```python
from build123d import *

# Parameters (mm, degrees)
MAIN_EXTRUSION_DEPTH         = 45
R_P_TITION_CIRCULAIRE1_DEPTH = 45
ESQUISSE2_R                  = 91.977766886
ESQUISSE2_R_2                = 40
GLOBAL_CIRCLE_DEPTH          = 1
CENTRAL_START                = 2
CENTRAL_FIXING_DEPTH         = 2
R_P_TITION_CIRCULAIRE2_COUNT = 8


# Read off the part's stored shape, not the designer's step: Répétition circulaire1
with BuildPart() as part:
    # Esquisse1 → Main Extrusion (new body)
    with BuildSketch(Plane.XY):
        with BuildLine():
            Line((57.667547326, 24.944747378), (84.602293038, 36.101484351))
            Line((84.602293038, 36.101484351), (85.750343335, 33.329845753))
            Line((85.750343335, 33.329845753), (58.815597623, 22.17310878))
            ThreePointArc((58.815597623, 22.17310878), (44, 0), (58.815597623, -22.17310878))
            Line((58.815597623, -22.17310878), (85.750343335, -33.329845753))
            Line((85.750343335, -33.329845753), (84.602293038, -36.101484351))
            Line((84.602293038, -36.101484351), (57.667547326, -24.944747378))
            ThreePointArc((57.667547326, -24.944747378), (41, 0), (57.667547326, 24.944747378))
        make_face()
    extrude(amount=MAIN_EXTRUSION_DEPTH)

    # Répétition circulaire1 outline → Répétition circulaire1 (add)
    with BuildSketch(Plane.XY):
        with BuildLine():
            Line((-84.202409209, -37.066889313), (-57.267663497, -25.91015234))
            ThreePointArc((-57.267663497, -25.91015234), (-31.112698372, -31.112698372), (-25.91015234, -57.267663497))
            Line((-25.91015234, -57.267663497), (-37.066889313, -84.202409209))
            Line((-37.066889313, -84.202409209), (-33.329845753, -85.750343335))
            Line((-33.329845753, -85.750343335), (-22.17310878, -58.815597623))
            ThreePointArc((-22.17310878, -58.815597623), (0, -44), (22.17310878, -58.815597623))
            Line((22.17310878, -58.815597623), (33.329845753, -85.750343335))
            Line((33.329845753, -85.750343335), (37.066889313, -84.202409209))
            Line((37.066889313, -84.202409209), (25.91015234, -57.267663497))
            ThreePointArc((25.91015234, -57.267663497), (31.112698372, -31.112698372), (57.267663497, -25.91015234))
            Line((57.267663497, -25.91015234), (84.202409209, -37.066889313))
            Line((84.202409209, -37.066889313), (84.602293038, -36.101484351))
            Line((84.602293038, -36.101484351), (57.667547326, -24.944747378))
            ThreePointArc((57.667547326, -24.944747378), (54.405305377, -23.327757675), (51.390283197, -21.286552275))
            ThreePointArc((51.390283197, -21.286552275), (28.991378029, -28.991378029), (21.286552275, -51.390283197))
            ThreePointArc((21.286552275, -51.390283197), (0, -41), (-21.286552275, -51.390283197))
            ThreePointArc((-21.286552275, -51.390283197), (-28.991378029, -28.991378029), (-51.390283197, -21.286552275))
            ThreePointArc((-51.390283197, -21.286552275), (-41, 0), (-51.390283197, 21.286552275))
            ThreePointArc((-51.390283197, 21.286552275), (-28.991378029, 28.991378029), (-21.286552275, 51.390283197))
            ThreePointArc((-21.286552275, 51.390283197), (0, 41), (21.286552275, 51.390283197))
            ThreePointArc((21.286552275, 51.390283197), (28.991378029, 28.991378029), (51.390283197, 21.286552275))
            ThreePointArc((51.390283197, 21.286552275), (54.405305377, 23.327757675), (57.667547326, 24.944747378))
            Line((57.667547326, 24.944747378), (84.602293038, 36.101484351))
            Line((84.602293038, 36.101484351), (84.202409209, 37.066889313))
            Line((84.202409209, 37.066889313), (57.267663497, 25.91015234))
            ThreePointArc((57.267663497, 25.91015234), (31.112698372, 31.112698372), (25.91015234, 57.267663497))
            Line((25.91015234, 57.267663497), (37.066889313, 84.202409209))
            Line((37.066889313, 84.202409209), (33.329845753, 85.750343335))
            Line((33.329845753, 85.750343335), (22.17310878, 58.815597623))
            ThreePointArc((22.17310878, 58.815597623), (0, 44), (-22.17310878, 58.815597623))
            Line((-22.17310878, 58.815597623), (-33.329845753, 85.750343335))
            Line((-33.329845753, 85.750343335), (-37.066889313, 84.202409209))
            Line((-37.066889313, 84.202409209), (-25.91015234, 57.267663497))
            ThreePointArc((-25.91015234, 57.267663497), (-31.112698372, 31.112698372), (-57.267663497, 25.91015234))
            Line((-57.267663497, 25.91015234), (-84.202409209, 37.066889313))
            Line((-84.202409209, 37.066889313), (-85.750343335, 33.329845753))
            Line((-85.750343335, 33.329845753), (-58.815597623, 22.17310878))
            ThreePointArc((-58.815597623, 22.17310878), (-44, 0), (-58.815597623, -22.17310878))
            Line((-58.815597623, -22.17310878), (-85.750343335, -33.329845753))
            Line((-85.750343335, -33.329845753), (-84.202409209, -37.066889313))
        make_face()
    extrude(amount=R_P_TITION_CIRCULAIRE1_DEPTH)

    # Esquisse2 → Global Circle (add)
    with BuildSketch(Plane.XY.offset(45)):
        with Locations(Location((0, 0, 0), (0, 0, 201.240037576))):
            Circle(ESQUISSE2_R)
        Circle(ESQUISSE2_R_2, mode=Mode.SUBTRACT)
    extrude(amount=GLOBAL_CIRCLE_DEPTH)

    # Esquisse3 → Central Fixing (add)
    with BuildSketch(Plane(origin=(0, 0, 45), x_dir=(-1, 0, 0), z_dir=(0, 0, -1)).offset(CENTRAL_START)):
        with BuildLine():
            Line((-5, 44.526610811), (-5, 0))
            Line((-5, 0), (-4, 0))
            Line((-4, 0), (-4, 5))
            Line((-4, 5), (4, 5))
            Line((4, 5), (4, 0))
            Line((4, 0), (5, 0))
            Line((5, 0), (5, 44.526610811))
            ThreePointArc((5, 44.526610811), (0, 44), (-5, 44.526610811))
        make_face()
    central_fixing = extrude(amount=-CENTRAL_FIXING_DEPTH)

    # Répétition circulaire2: Central Fixing ×8 about axis
    r_p_tition_circulaire2_axis = Axis((0, 0, 0), (0, 0, 1))
    for i in range(1, R_P_TITION_CIRCULAIRE2_COUNT):
        add(central_fixing.rotate(r_p_tition_circulaire2_axis, i * 360 / R_P_TITION_CIRCULAIRE2_COUNT))


solid = part.part
```
The model under review builds one solid part; all positions refer to its coordinate system, in mm. A direction names the side the tool comes from. Round coordinates to 2 decimals unless told otherwise and drop trailing zeros. Loops run counter-clockwise (first coordinate to the right, second up) from the corner with the lowest first, then second, coordinate; pieces in that order, holes last. Notation, with made-up numbers: (-20.5, 4) - (-4.5, 4) arc R19 cw to (-4.5, 9) - close; hole circle Ø5 at (71.5, 68.5). An arc over 180 degrees is marked (long way). Use a Markdown table: item, result. Add a question column.
Q1. For probe 1 along Y at (x, z) = (0, 45.45); probe 2 along Y at (x, z) = (-30.5, 35); probe 3 along Y at (x, z) = (35, 24), list the stretches that pass through material, from the lowest coordinate up.
Q2. Add section C-C (y = -75). State the section outline as (x, z) points.
Q3. Machinability: for faces 1 (the face through (0, -44, 22)), 2 (the face through (-70.55, 31.41, 22.18)), 3 (the face through (30.84, 31.39, 22.18)), 4 (the face through (31.41, 70.55, 22.18)), which of the approach directions +Z, -Z, +X, -X, +Y, -Y give a long, thin tool a straight path to every point of the face, cutting with its end or side? Answer none if there is none.
Q4. The part is to be moulded in two halves that separate along X. For faces 5 (the face through (44, 0, 22)), 6 (the face through (0, -41, 22)), 7 (the face through (-72.47, 27.83, 22.18)), 8 (the face through (-18, -40, 45)), say which applies: pulls with the +X half, pulls with the -X half, needs draft (parallel to the pull), parting line crosses it, or undercut.
Q5. Add section B-B (y = 9.5). State the section outline as (x, z) points.
Q6. Insertion check: pin 1 Ø4 at (y, z) = (-57.5, 36) entering from -X; pin 2 Ø1.5 at (x, y) = (49.5, -66.5) entering from -Z; pin 3 Ø2 at (y, z) = (-32, 43.5) entering from -X. Each pin has a flat end and moves straight along its axis. Give the tip position at first contact, or say it passes through.
Q7. Add section D-D (x = -73). State the section outline as (y, z) points, plus the area to 3 significant figures.
Q8. Add section A-A (x = -7.5). State the section outline as (y, z) points, plus the area to 3 significant figures.
Worked answers:
| question | item | result |
|---|---|---|
| 1 | probe 1 | -91.98 to -40, 40 to 91.98 |
| 1 | probe 2 | -78.92 to -68.35, -31.75 to -27.59, 27.59 to 31.75, 68.35 to 78.92 |
| 1 | probe 3 | -85.06 to -79.21, -27.96 to -24.46, 24.46 to 27.96, 79.21 to 85.06 |
| 2 | outline | (-53.24, 45) - (-33.26, 45) - (-33.26, 0) - (-28.88, 0) - (-28.88, 45) - (28.88, 45) - (28.88, 0) - (33.26, 0) - (33.26, 45) - (53.24, 45) - (53.24, 46) - (-53.24, 46) - close |
| 3 | face 1 | -Z, -Y |
| 3 | face 2 | -Z, +Y |
| 3 | face 3 | -Z |
| 3 | face 4 | -Z, +X |
| 4 | face 5 | pulls with the +X half |
| 4 | face 6 | undercut |
| 4 | face 7 | pulls with the -X half |
| 4 | face 8 | undercut |
| 5 | outline | (-91.49, 45) - (-45.96, 45) - (-45.96, 0) - (-42.73, 0) - (-42.73, 45) - (-38.86, 45) - (-38.86, 46) - (-91.49, 46) - close; (-16.57, 43) - (16.57, 43) - (16.57, 45) - (-16.57, 45) - close; (38.86, 45) - (42.73, 45) - (42.73, 0) - (45.96, 0) - (45.96, 45) - (91.49, 45) - (91.49, 46) - (38.86, 46) - close |
| 6 | pin 1 | x = -26.83 |
| 6 | pin 2 | z = 45 |
| 6 | pin 3 | x = -84.95 |
| 7 | outline | (-55.95, 45) - (-32.43, 45) - (-32.43, 0) - (-28.05, 0) - (-28.05, 45) - (28.05, 45) - (28.05, 0) - (32.43, 0) - (32.43, 45) - (55.95, 45) - (55.95, 46) - (-55.95, 46) - close |
| 7 | area | 506 mm² |
| 8 | outline | (-91.67, 45) - (-45.2, 45) - (-45.2, 0) - (-42.06, 0) - (-42.06, 45) - (-39.29, 45) - (-39.29, 46) - (-91.67, 46) - close; (-14.57, 43) - (14.57, 43) - (14.57, 45) - (-14.57, 45) - close; (39.29, 45) - (42.06, 45) - (42.06, 0) - (45.2, 0) - (45.2, 45) - (91.67, 45) - (91.67, 46) - (39.29, 46) - close |
| 8 | area | 446 mm² |
